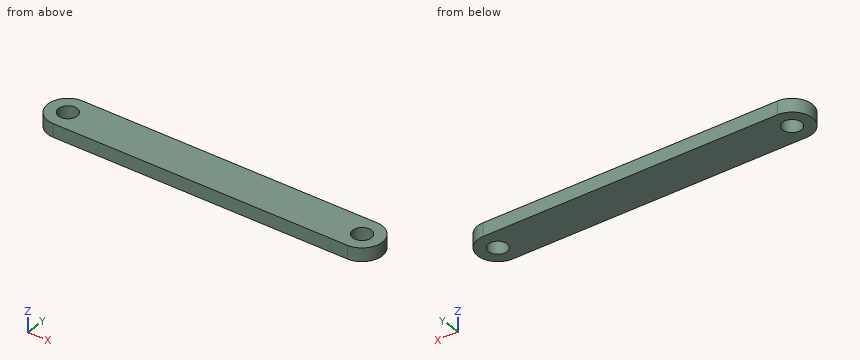
```python
from build123d import *

# Parameters (mm, degrees)
BOSS_EXTRUDE1_DEPTH = 2.54
SKETCH2_R           = 1.778
CUT_EXTRUDE1_DEPTH  = 2.54


with BuildPart() as part:
    # Sketch1 → Boss-Extrude1 (new body)
    with BuildSketch(Plane.XY):
        with BuildLine():
            Line((-27.94, 0), (27.94, 0))
            ThreePointArc((27.94, 0), (31.75, -3.81), (27.94, -7.62))
            Line((27.94, -7.62), (-27.94, -7.62))
            ThreePointArc((-27.94, -7.62), (-31.75, -3.81), (-27.94, 0))
        make_face()
    extrude(amount=BOSS_EXTRUDE1_DEPTH)

    # Sketch2 → Cut-Extrude1 (cut)
    with BuildSketch(Plane.XY.offset(2.54)):
        with Locations((-27.94, -3.81)):
            Circle(SKETCH2_R)
    cut_extrude1 = extrude(amount=-CUT_EXTRUDE1_DEPTH, mode=Mode.SUBTRACT)

    # Mirror1: Cut-Extrude1 across plane
    add(cut_extrude1.mirror(Plane(origin=(0, 0, 0), x_dir=(0, 0, 1), z_dir=(1, 0, 0))), mode=Mode.SUBTRACT)


solid = part.part
```
Source: CAD feature listing. Evaluate the final solid. Frame: model axes, mm. Give positions to 0.01 mm unless a question says otherwise; leave off trailing zeros. Loops run counter-clockwise (first coordinate to the right, second up) from the corner with the lowest first, then second, coordinate; pieces in that order, holes last. Notation, with made-up numbers: M 89,-33.75 L 104,-33.75 A15 ccw 104,-22.75 Z; hole C 50.5,24 d11. An arc over 180 degrees is marked long. Put each result on its own line as item: value.
Q1. Section A-A (y = -3.81). Return the cut outline in (x, z).
Response values:
outline: M -31.75,0 L -29.72,0 L -29.72,2.54 L -31.75,2.54 Z; M -26.16,0 L 26.16,0 L 26.16,2.54 L -26.16,2.54 Z; M 29.72,0 L 31.75,0 L 31.75,2.54 L 29.72,2.54 Z
Q2. Section B-B (z = 1.05). Return the cut outline in (x, y), and give its area (3 significant figures).
Response values:
outline: M -27.94,-7.62 L 27.94,-7.62 A3.81 ccw 27.94,0 L -27.94,0 A3.81 ccw Z; hole C -27.94,-3.81 d3.56; hole C 27.94,-3.81 d3.56
area: 452 mm²
Q3. Line query: probe 1 along Y at (x, z) = (27.94, 1.65); probe 2 along X at (y, z) = (-1.5, 0.35); probe 3 along X at (y, z) = (-7.25, 0.4). Output: solid intervals per line, ascending. Write a range as [from, to].
Response values:
probe 1: y = [-7.62, -5.59], [-2.03, 0]
probe 2: x = [-30.97, 30.97]
probe 3: x = [-29.58, 29.58]
Q4. Section D-D (y = -6.5). Return the cut outline in (x, z).
Response values:
outline: M -30.64,0 L 30.64,0 L 30.64,2.54 L -30.64,2.54 Z
Q5. Section C-C (y = -1). Return the cut outline in (x, z).
Response values:
outline: M -30.51,0 L 30.51,0 L 30.51,2.54 L -30.51,2.54 Z
